```python
from build123d import *

# Parameters (mm, degrees)
SKETCH1_R           = 7.5
SKETCH1_R_2         = 5
BOSS_EXTRUDE1_DEPTH = 5
SKETCH2_W           = 5
SKETCH2_H           = 15
BOSS_EXTRUDE2_DEPTH = 50
SKETCH3_W           = 5
SKETCH3_H           = 15
BOSS_EXTRUDE3_DEPTH = 20
SKETCH4_R           = 5
CUT_EXTRUDE1_DEPTH  = 15
FILLET1_R           = 7.5
CHAMFER1_SIZE       = 5
CUT_EXTRUDE2_DEPTH  = 5
CHAMFER2_SIZE       = 1.5
CHAMFER3_SIZE       = 2.5
CHAMFER4_SIZE       = 2.5
SKETCH10_R          = 1.75
CUT_EXTRUDE4_DEPTH  = 10


with BuildPart() as part:
    # Sketch1 → Boss-Extrude1 (new body)
    # profile 1 of 2: a face of its own
    with BuildSketch(Plane.XY):
        Circle(SKETCH1_R)
        Circle(SKETCH1_R_2, mode=Mode.SUBTRACT)
    # profile 2 of 2: a face of its own
    with BuildSketch(Plane.XY):
        with BuildLine():
            Line((15, 7.5), (0, 7.5))
            ThreePointArc((0, 7.5), (5.303300859, 5.303300859), (7.5, 0))
            ThreePointArc((7.5, 0), (5.303300859, -5.303300859), (0, -7.5))
            Line((0, -7.5), (15, -7.5))
            Line((15, -7.5), (15, 7.5))
        make_face()
    extrude(amount=BOSS_EXTRUDE1_DEPTH)

    # Sketch2 → Boss-Extrude2 (add)
    with BuildSketch(Plane.XY.offset(5)):
        with Locations((12.5, 0)):
            Rectangle(SKETCH2_W, SKETCH2_H)
    extrude(amount=BOSS_EXTRUDE2_DEPTH)

    # Sketch3 → Boss-Extrude3 (add)
    with BuildSketch(Plane(origin=(15, 0, 0), x_dir=(0, 0, -1), z_dir=(1, 0, 0))):
        with Locations((-52.5, 0)):
            Rectangle(SKETCH3_W, SKETCH3_H)
    extrude(amount=BOSS_EXTRUDE3_DEPTH)

    # Sketch4 → Cut-Extrude1 (cut)
    with BuildSketch(Plane(origin=(0, 0, 50), x_dir=(-1, 0, 0), z_dir=(0, 0, -1))):
        with Locations(Location((-27.5, 0, 0), (0, 0, 90))):
            Circle(SKETCH4_R)
    extrude(amount=-CUT_EXTRUDE1_DEPTH, mode=Mode.SUBTRACT)

    # Fillet1
    fillet1_edges = [part.edges().sort_by_distance(p)[0] for p in [
        (35, -7.5, 52.5),
        (35, 7.5, 52.5),
    ]]
    fillet(fillet1_edges, radius=FILLET1_R - 0.0001)  # a hair under: the kernel refuses the full size

    # Chamfer1
    chamfer1_edges = [part.edges().sort_by_distance(p)[0] for p in [
        (10, 0, 55),
        (15, 0, 0),
    ]]
    chamfer(chamfer1_edges, length=CHAMFER1_SIZE)

    # Sketch5 → Cut-Extrude2 (cut)
    with BuildSketch(Plane.ZY.offset(-10)):
        Polygon((10, -7.5), (13, -4.5), (42, -4.5), (45, -7.5), align=None)
        Polygon((45, 7.5), (10, 7.5), (13, 4.5), (42, 4.5), align=None)
    extrude(amount=-CUT_EXTRUDE2_DEPTH, mode=Mode.SUBTRACT)

    # Chamfer2
    chamfer2_edges = [part.edges().sort_by_distance(p)[0] for p in [
        (15, -4.5, 27.5),
        (10, -4.5, 27.5),
        (15, 4.5, 27.5),
        (10, 4.5, 27.5),
    ]]
    chamfer(chamfer2_edges, length=CHAMFER2_SIZE)

    # Chamfer3
    chamfer3_edges = [part.edges().sort_by_distance(p)[0] for p in [
        (10, 7.5, 47.5),
        (12.5, 7.5, 52.5),
        (12.5, 7.5, 2.5),
        (10, -7.5, 47.5),
        (12.5, -7.5, 52.5),
        (12.5, -7.5, 2.5),
        (15, 7.5, 7.5),
        (15, -7.5, 7.5),
        (15, -5.25, 12.25),
        (10, -5.25, 42.75),
        (15, 5.25, 12.25),
        (10, 5.25, 42.75),
    ]]
    chamfer(chamfer3_edges, length=CHAMFER3_SIZE)

    # Chamfer4
    chamfer4_edges = [part.edges().sort_by_distance(p)[0] for p in [
        (10, 0, 5),
        (15, 0, 50),
    ]]
    chamfer(chamfer4_edges, length=CHAMFER4_SIZE)

    # Sketch10 → Cut-Extrude4 (cut)
    with BuildSketch(Plane(origin=(15, 0, 0), x_dir=(0, 0, -1), z_dir=(1, 0, 0))):
        with Locations((-25.732233047, 0)):
            Circle(SKETCH10_R)
        with Locations((-18.232233047, 0)):
            Circle(SKETCH10_R)
        with Locations(Location((-33.232233047, 0, 0), (0, 0, 90))):
            Circle(SKETCH10_R)
    extrude(amount=-CUT_EXTRUDE4_DEPTH, mode=Mode.SUBTRACT)


solid = part.part
```
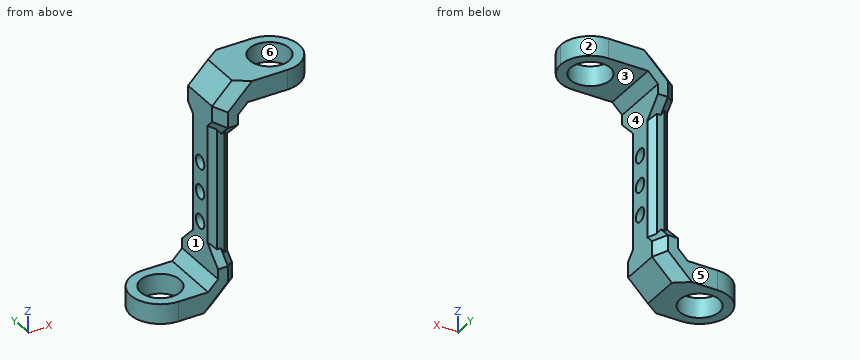
Input: part model. Units: mm. Frame: model coordinates. Face numbers are marked on the shaded views. A direction names the side the tool comes from. Give positions to 0.01 mm unless a question says otherwise; leave off trailing zeros. Order: outer loops, then holes, each group sorted by start corner. A loop starts at its lowest first (then second) coordinate and runs counter-clockwise, first axis right, second up. Notation, with made-up numbers: (-27.5, 51.5) - (19.5, 51.5) arc R12 ccw to (19.5, 71.5) - close; hole circle Ø10 at (59, 72.5). An arc over 180 degrees is marked (long way). Use a Markdown table: item, result.
(1) Section query A-A (y = 3.75). Output: boundary loops of the cut face in (x, z), then the cut area to 3 significant figures.
Computed values:
| item | result |
|---|---|
| outline | (-6.5, 0) - (-3.31, 0) - (-3.31, 5) - (-6.5, 5) - close; (3.31, 0) - (10, 0) - (15, 5) - (15, 10.21) - (14.25, 11.28) - (14.25, 41.25) - (15, 41.25) - (15, 47.5) - (17.5, 50) - (24.19, 50) - (24.19, 55) - (15, 55) - (10, 50) - (10, 44.79) - (10.75, 43.72) - (10.75, 13.75) - (10, 13.75) - (10, 7.5) - (7.5, 5) - (3.31, 5) - close; (30.81, 50) - (34, 50) - (34, 55) - (30.81, 55) - close |
| area | 322 mm2 |
(2) Pin query (flat end, axial travel): pin 1 (3 mm diameter, centred on y = 0, z = 18.23, fed in from -X); pin 2 (8 mm diameter, centred on x = 24, y = -1.5, fed in from -Z); pin 3 (4 mm diameter, centred on y = 0, z = 33.23, fed in from +X); pin 4 (0.6 mm diameter, centred on x = 13, z = 19.5, fed in from +Y). Return the tip coordinate at first contact, or that it passes through.
Computed values:
| item | result |
|---|---|
| pin 1 | passes through |
| pin 2 | stops at z = 50 |
| pin 3 | stops at x = 15 |
| pin 4 | stops at y = 4.5 |
(3) Section query C-C (x = 26). Output: boundary loops of the cut face in (y, z), then the cut area to 3 significant figures.
Computed values:
| item | result |
|---|---|
| outline | (-7.5, 50) - (-4.77, 50) - (-4.77, 55) - (-7.5, 55) - close; (4.77, 50) - (7.5, 50) - (7.5, 55) - (4.77, 55) - close |
| area | 27.3 mm2 |
(4) Line query: line 1 (Z direction, x = 7, y = -3); line 2 (Y direction, x = 27, z = 52); line 3 (Z direction, x = 26, y = 5.5). Output: solid intervals per line, ascending. Write a range as from..to.
Computed values:
| item | result |
|---|---|
| line 1 | z = 0..5 |
| line 2 | y = -7.5..-4.97, 4.97..7.5 |
| line 3 | z = 50..55 |
(5) Draft query along X for the marked faces 4, 5 and 6. Return one class per face: released by +X, released by -X, zero draft, split by the parting line, or undercut.
Computed values:
| item | result |
|---|---|
| face 4 | released by +X |
| face 5 | zero draft |
| face 6 | undercut |
(6) Access query for the marked faces 1, 2 and 3. Directions: +Z, -Z, +X, -X, +Y, -Y. A direction counts if a zero-diameter tool reaches every point of the face in a straight line with its end or side. Return the directions, or none.
Computed values:
| item | result |
|---|---|
| face 1 | +Z, -X, +Y, -Y |
| face 2 | +Z, -Z, +X, +Y |
| face 3 | -Z, +X, +Y, -Y |
(7) Section query D-D (x = 19.5). Output: boundary loops of the cut face in (y, z).
Computed values:
| item | result |
|---|---|
| outline | (-7.5, 50) - (7.5, 50) - (7.5, 55) - (-7.5, 55) - close |
(8) Section query B-B (z = 36). Output: boundary loops of the cut face in (x, y), then the cut area to 3 significant figures.
Computed values:
| item | result |
|---|---|
| outline | (10, -3) - (11.5, -4.5) - (13.5, -4.5) - (15, -3) - (15, 3) - (13.5, 4.5) - (11.5, 4.5) - (10, 3) - close |
| area | 40.5 mm2 |
